Autodesk Inventor part; units mm, degrees
ref_plane "Work Plane1" through (-18.2456, 0, 0) normal (0, -0.8660254, -0.5) x (1, 0, 0)
ref_plane "YZ Plane" through (0, 0, 0) normal (1, 0, 0) x (0, 1, 0)
ref_plane "XZ Plane" through (0, 0, 0) normal (0, 1, 0) x (-1, 0, 0)
sketch "Skizze1" plane through (0, 0, 0) normal (1, 0, 0) x (0, 1, 0)
  line L0 (-10.3923, 0) -> (-5.1962, 9)
  line L1 (-5.1962, 9) -> (5.1962, 9)
  line L2 (5.1962, 9) -> (10.3923, 0)
  line L3 (10.3923, 0) -> (5.1962, -9)
  line L4 (5.1962, -9) -> (-5.1962, -9)
  line L5 (-5.1962, -9) -> (-10.3923, 0)
  point P0 (0, 0)
  point P1 (0, 0)
  dimension "d0" = 20.7846
extrude "Körper" add sketch "Skizze1" along normal blind 12
sketch "Skizze2" plane through (0, 0, 0) normal (0, 0, 1) x (1, 0, 0)
  line L0 (0, 5.1962) -> (0, 10.3923)
  line L1 (0, 10.3923) -> (12, 10.3923)
  line L2 (12, 5.1962) -> (12, 10.3923)
  line L3 (-2.4, 0) -> (14.4, 0)
  line L4 (1.1993, 10.3923) -> (0, 8.315)
  line L5 (10.8007, 10.3923) -> (12, 8.315)
  dimension "d3" = 30
  dimension "d4" = 30
  dimension "d5" = 16.63
  dimension "d6" = 16.63
revolve "Fase1" cut sketch "Skizze2" angle 360 about axis through (-10, 0, 0) along (1, 0, 0)
sketch "Skizze3" plane through (12, 0, 0) normal (1, 0, 0) x (0, 0, -1)
  arc A0 (-0.625, -1.0825) -> (0.625, -1.0825) centre (0, 0) ccw
hole "Gewinde" at (12, 0, 0) direction (-1, 0, 0) diameter 10.376 end through all
chamfer "Fase2" distance 0.8119 angle 30 1 edges at (12, 0, 5.188) measured on face at (12, 7.1795, -0.8718)
chamfer "Fase3" distance 0.8119 angle 30 1 edges at (0, 0, 5.188) measured on face at (0, 7.1795, -0.8718)
ref_plane "Work Plane1" through (-18.2456, 0, 0) normal (0, -0.8660254, -0.5) x (1, 0, 0)
equation "\"d0\" = 1.1547 * SW"
equation "\"d1\" = KOH"
equation "\"d3\" = ANG1"
equation "\"d4\" = ANG2"
equation "\"d5\" = SW0"
equation "\"d6\" = SW01"
equation "\"d8\" = -0.5 * GD1 + 0.5 * NND"
equation "\"d40\" = -0.5 * GD1 + 0.5 * NND"
equation "\"d10\" = -0.5 * GD1 + 0.5 * NND"
equation "\"d41\" = -0.5 * GD1 + 0.5 * NND"
equation "\"ANG1\" = 30deg"
equation "\"ANG2\" = 30deg"
equation "\"NND\" = 12"
equation "\"KOH\" = 12"
equation "\"SW\" = 18"
equation "\"SW0\" = 16.63"
equation "\"SW01\" = SW0"
equation "\"GUL\" = 0.541266 * PTC"
equation "\"THREADDIA\" = 12"
equation "\"TOA\" = 30deg"
equation "\"PTC\" = 1.5"
equation "\"E0\" = 20.03"
equation "\"GAL\" = 0.541266 * PTC"
equation "\"KOH1\" = 9.26"
properties part number "ISO 8674 - M12 x 1,5" material "Stahl"
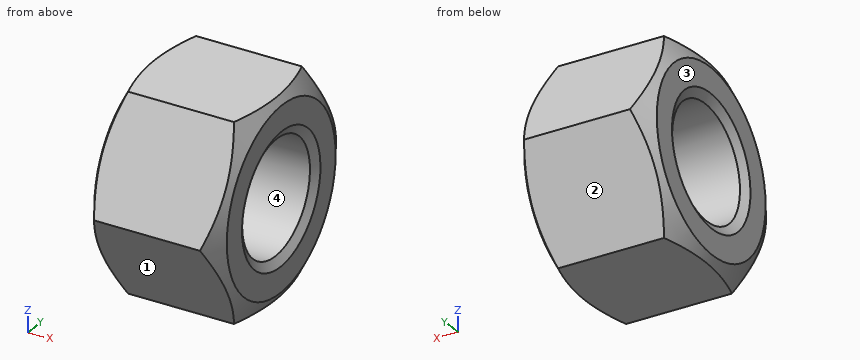
Work out the finished part from the listing and answer in its coordinate system (mm). Face numbers are marked on the shaded views. Coordinates: 2 decimals unless noted, no trailing zeros. Order: outer loops, then holes, each group sorted by start corner. A loop starts at its lowest first (then second) coordinate and runs counter-clockwise, first axis right, second up. Notation, with made-up numbers: M -16.75,67 L -5.75,67 A19 cw -5.75,91 Z; hole C -20,80 d9. An arc over 180 degrees is marked long. Use CSV: the item, a comma, the result in double quotes.
1) Consider line 1 (Z direction, x = 8.75, y = 0); line 2 (Y direction, x = 4, z = -3.5); line 3 (Z direction, x = 10.5, y = -1.75). Determine where each line is inside the solid, lowest interval first. Write a range as [from, to].
Worked out:
line 1,"z = [-9, -5.19], [5.19, 9]"
line 2,"y = [-8.37, -3.83], [3.83, 8.37]"
line 3,"z = [-9, -4.88], [4.88, 9]"
2) Section B-B on x = 3.5 is taken. Write down the section's boundary in (y, z).
Worked out:
outline,"M -10.39,0 L -5.2,-9 L 5.2,-9 L 10.39,0 L 5.2,9 L -5.2,9 Z; hole C 0,0 d10.38"
3) Flat-ended cylindrical pins translate along their axes: pin 1 Ø2 at (x, z) = (10.5, 5) entering from +Y; pin 2 Ø6 at (x, z) = (1.5, 6.5) entering from +Y; pin 3 Ø3 at (x, z) = (4.5, -4) entering from -Y. Find the tip coordinate at first contact, or state that the pin passes through.
Worked out:
pin 1,"stops at y = 8.08"
pin 2,"stops at y = 8.37"
pin 3,"stops at y = -8.95"
4) Section A-A on y = 0 is taken. Write down the section's boundary in (x, z) (3 decimals), plus the area to 3 significant figures.
Worked out:
outline,"M 0,-8.315 L 0.395,-9 L 11.605,-9 L 12,-8.315 L 12,-6 L 11.531,-5.188 L 0.469,-5.188 L 0,-6 Z; M 0,6 L 0.469,5.188 L 11.531,5.188 L 12,6 L 12,8.315 L 11.605,9 L 0.395,9 L 0,8.315 Z"
area,"90.2 mm^2"
5) Determine the mould class of the marked faces 1, 2, 3 and 4 for opening direction Y: released by +Y, released by -Y, zero draft, split by the parting line, or undercut.
Worked out:
face 1,"released by -Y"
face 2,"released by +Y"
face 3,"zero draft"
face 4,"undercut"
